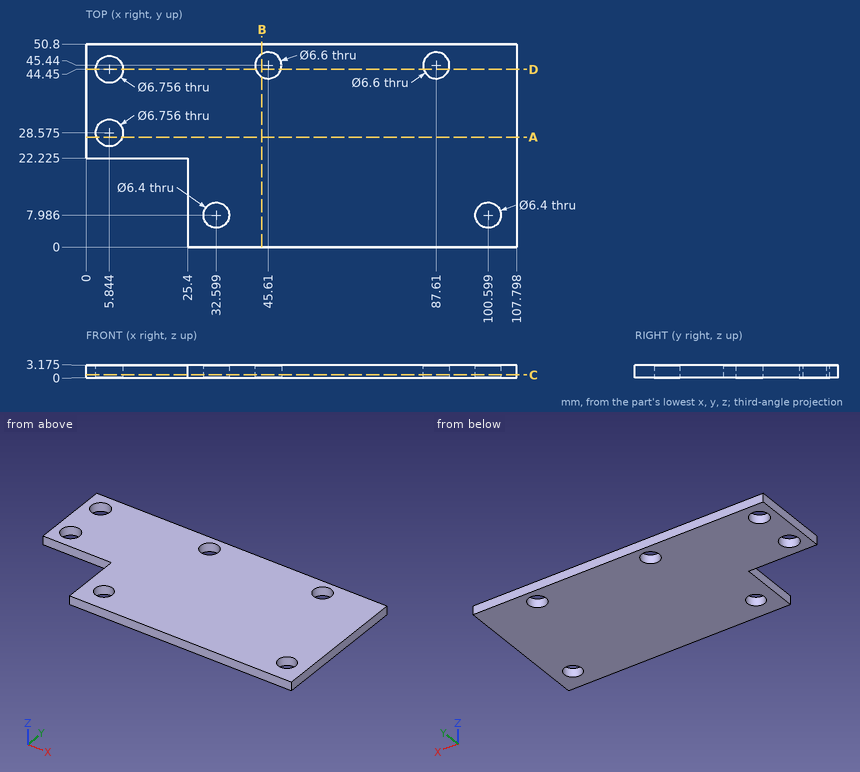
Input: dimensioned drawing with shaded views. Units: mm. Origin: part minimum x, y, z. Give positions to 0.01 mm unless a question says otherwise; leave off trailing zeros. Write each loop counter-clockwise with the first axis right and the second up, starting at its lowest first coordinate (ties: lowest second). Pieces come first, ordered by that corner, then holes. Notation, with made-up numbers: (7, 16) -> (59, 16) arc R16 ccw to (59, 22) -> close; hole circle Ø7 at (43, 20.25). An arc over 180 degrees is marked (long way). Answer as a JSON object with one key per item and string values.
1. Cut plane B-B on x = 44. Output: boundary loops of the cut face in (y, z) (1 decimal).
Ans:
{"outline": "(0, 0) -> (42.6, 0) -> (42.6, 3.2) -> (0, 3.2) -> close; (48.3, 0) -> (50.8, 0) -> (50.8, 3.2) -> (48.3, 3.2) -> close"}
2. Cut plane D-D on y = 44.45. Output: boundary loops of the cut face in (x, z) (1 decimal).
Ans:
{"outline": "(0, 0) -> (2.5, 0) -> (2.5, 3.2) -> (0, 3.2) -> close; (9.2, 0) -> (42.5, 0) -> (42.5, 3.2) -> (9.2, 3.2) -> close; (48.8, 0) -> (84.5, 0) -> (84.5, 3.2) -> (48.8, 3.2) -> close; (90.8, 0) -> (107.8, 0) -> (107.8, 3.2) -> (90.8, 3.2) -> close"}
3. Cut plane A-A on y = 27.5. Output: boundary loops of the cut face in (x, z) (1 decimal), and give its area (3 significant figures).
Ans:
{"outline": "(0, 0) -> (2.6, 0) -> (2.6, 3.2) -> (0, 3.2) -> close; (9, 0) -> (107.8, 0) -> (107.8, 3.2) -> (9, 3.2) -> close", "area": "322 mm^2"}
4. Cut plane C-C on z = 0.75. Count the separate pieces of the cut face and the enclosed holes in it, and give its area (3 significant figures).
Ans:
{"separate pieces": "1", "enclosed holes": "6", "area": "4,710 mm^2"}
5. Ray query, probe 1 along Y at (x, z) = (46, 1.1); probe 2 along X at (y, z) = (10, 0.8) (1 decimal); probe 3 along Y at (x, z) = (9.5, 1.25) (1 decimal). Return the intervals inside material, ascending. Write a range as from..to.
Ans:
{"probe 1": "y = 0..42.16, 48.72..50.8", "probe 2": "x = 25.4..30.1, 35.1..98.1, 103.1..107.8", "probe 3": "y = 22.2..50.8"}
6. Contact query for a flat-ended pin moving along its axis: pin 1 (1 mm diameter, centred on x = 8.5, z = 1.5, fed in from -Y) (3 decimals). Output: stop coordinate, or through.
Ans:
{"pin 1": "stops at y = 22.225"}
